The model under review builds one solid part; all positions refer to its coordinate system, in mm. A direction names the side the tool comes from. Coordinates: 2 decimals unless noted, no trailing zeros. Order: outer loops, then holes, each group sorted by start corner. A loop starts at its lowest first (then second) coordinate and runs counter-clockwise, first axis right, second up. Notation, with made-up numbers: M 80.5,79.5 L 127.5,79.5 A22 ccw 127.5,101.5 Z; hole C 30,86.25 d2. An arc over 180 degrees is marked long. One line per item, written item: value.
Solid Edge part; units mm, degrees
sketch "Sketch1" plane through (0, 0, 0) normal (0, 0, 1) x (1, 0, 0)
  line L0 (0, 7.5) -> (0, -7.5)
  line L1 (0, -7.5) -> (4, -7.5)
  line L2 (4, -7.5) -> (4, -4)
  line L3 (4, -4) -> (6, -4)
  line L4 (6, -4) -> (6, 4)
  line L5 (6, 4) -> (4, 4)
  line L6 (4, 4) -> (4, 7.5)
  line L7 (4, 7.5) -> (0, 7.5)
  dimension "D1" = 6
  dimension "D2" = 4
  dimension "D3" = 6
extrude "Protrusion1" add sketch "Sketch1" along normal mid plane 6
sketch "Sketch2" plane through (2, -7.5, 0) normal (0, -1, 0) x (1, 0, 0)
  line L0 (-2, -1.5) -> (-2, 1.5)
  line L1 (-2, 1.5) -> (-0.5, 0)
  line L2 (-0.5, 0) -> (-2, -1.5)
  dimension "D1" = 2
extrude "Cutout1" cut sketch "Sketch2" against normal up to next
sketch "Sketch3" plane through (6, 0, 3) normal (0, 0, 1) x (1, 0, 0)
  line L0 (-6, 1.5) -> (-4.5, 0)
  line L1 (-4.5, 0) -> (-6, -1.5)
  line L2 (-6, -1.5) -> (-6, 1.5)
  dimension "D1" = 6
extrude "Cutout2" cut sketch "Sketch3" against normal through all
chamfer "Chamfer_1" distance 1.5 angle 45 2 edges at (4, -4, 0) (4, 4, 0)
properties material "Polyethylene, low density"
(1) Mouldability with a two-part tool opening along Y and no side actions: class faces 6 (the flat face through (4.7, -4.8, 0)), 7 (the flat face through (0.8, -0.7, 1.9)), 8 (the flat face through (0, 5, 2)) as +Y half, -Y half, draft (parallel to the pull), parting line (faces both ways), or undercut.
Geometry results:
face 6: -Y half
face 7: undercut
face 8: draft
(2) We need section C-C, the plane z = -0.85. State the section outline as (x, y) points, plus the area to 3 significant figures.
Geometry results:
outline: M 0.65,-7.5 L 4,-7.5 L 4,-5.5 L 5.5,-4 L 6,-4 L 6,4 L 5.5,4 L 4,5.5 L 4,7.5 L 0.65,7.5 L 0.65,0.85 L 1.5,0 L 0.65,-0.85 Z
area: 67.8 mm2
(3) We need section A-A, the plane z = -0.2. State the section outline as (x, y) points, plus the area to 3 significant figures.
Geometry results:
outline: M 1.3,-7.5 L 4,-7.5 L 4,-5.5 L 5.5,-4 L 6,-4 L 6,4 L 5.5,4 L 4,5.5 L 4,7.5 L 1.3,7.5 L 1.3,0.2 L 1.5,0 L 1.3,-0.2 Z
area: 58.7 mm2
(4) For L1, parallel to Y at x = 0.35, z = -2.2; L2, parallel to Y at x = 1.3, z = 1.65; L3, parallel to Z at x = 1.4, y = 2.25, list the stretches that pass through material, from the lowest coordinate up.
Geometry results:
L1: y = -7.5 to -1.15, 1.15 to 7.5
L2: y = -7.5 to -0.2, 0.2 to 7.5
L3: z = -3 to -0.1, 0.1 to 3
(5) Tool access review of faces 1 (the flat face through (0.7, 0.8, -1.8)), 2 (the flat face through (4, -7, 0)), 3 (the flat face through (0.7, -3.8, 0.8)), 4 (the flat face through (4, 6, 0)), 5 (the flat face through (0, 5, -2)): name each direction out of +Z, -Z, +X, -X, +Y, -Y from which nothing blocks a thin tool from reaching the whole face with its end or side.
Geometry results:
face 1: +Z, -Z, -X
face 2: +Z, -Z, +X, -Y
face 3: -X, +Y, -Y
face 4: +Z, -Z, +X, +Y
face 5: +Z, -Z, -X, +Y, -Y
(6) We need section D-D, the plane x = 5.25. State the section outline as (y, z) points, plus the area to 3 significant figures.
Geometry results:
outline: M -4.25,-3 L 4.25,-3 L 4.25,3 L -4.25,3 Z
area: 51.0 mm2
(7) We need section B-B, the plane y = 0.25. State the section outline as (x, z) points, plus the area to 3 significant figures.
Geometry results:
outline: M 1.25,-3 L 6,-3 L 6,3 L 1.25,3 L 1.25,0.25 L 1.5,0 L 1.25,-0.25 Z
area: 28.4 mm2
(8) Insertion check: pin 1 Ø2 at (y, z) = (-7, 1) entering from +X. The pin has a flat end and moves straight along its axis. Give the tip position at first contact, or say it passes through.
Geometry results:
pin 1: stops at x = 4
